Autodesk Inventor part; units mm, degrees
ref_plane "YZ Plane" through (0, 0, 0) normal (1, 0, 0) x (0, 1, 0)
ref_plane "XZ Plane" through (0, 0, 0) normal (0, 1, 0) x (-1, 0, 0)
ref_plane "XY Plane" through (0, 0, 0) normal (0, 0, 1) x (1, 0, 0)
sketch "Sketch1" plane through (0, 0, 0) normal (0, 0, 1) x (1, 0, 0)
  line L0 (0, 0) -> (10, 0)
  line L1 (10, 0) -> (10, 48.3509)
  line L2 (10, 48.3509) -> (59.1053, 20)
  line L3 (59.1053, 20) -> (59.1053, 60)
  line L4 (59.1053, 60) -> (23.094, 60)
  line L5 (23.094, 60) -> (0, 100)
  line L6 (0, 100) -> (0, 0)
  dimension "d0" = 20
  dimension "d1" = 30
  dimension "d2" = 100
  dimension "d3" = 60
  dimension "d4" = 40
  dimension "d5" = 118.2105
  dimension "d6" = 60
revolve "Revolution1" add sketch "Sketch1" angle 360 about axis through (0, 100, 0) along (0, -1, 0)
fillet "Fillet1" radius 20 1 edges at (-10, 48.3509, 0)
equation "\"ITERACOES\" = 0"
equation "\"VALORES_OTIMOS\" = 118.21054"
properties part number "Mass_otimization" material "Steel, Mild"
Could you check a few things on this model? Use its own coordinates, in mm. A direction names the side the tool comes from. Give positions to 0.01 mm unless a question says otherwise; leave off trailing zeros. Order: outer loops, then holes, each group sorted by start corner. A loop starts at its lowest first (then second) coordinate and runs counter-clockwise, first axis right, second up. Notation, with made-up numbers: (13.5, -39) -> (23.5, -39) arc R8 cw to (23.5, -25) -> close; hole circle Ø3 at (-17, 30.25). An arc over 180 degrees is marked (long way). Answer in a Markdown table with one row per item. Add a question column.
Item 1: I'm going to push flat-ended pins straight in: P1, Ø3, axis at x = 38.5, y = 24.5, coming from the +Z side; P2, Ø8, axis at y = 58, z = 15, coming from the -X side; P3, Ø10, axis at y = 34, z = 44.5, coming from the +X side. Where does each tip first touch, or does it pass through?
Item 2: Please list where these lines run through material, in increasing order: probe 1 along Z at (x, y) = (-7.5, 29); probe 2 along Z at (x, y) = (-4, 23); probe 3 along X at (y, z) = (23, 5.5).
Item 3: Imagine slicing it at A-A (y = 47). List the corners of the cut face in (x, z) for me, and give its area (3 significant figures).
Item 4: Imagine slicing it at B-B (y = 68.5). List the corners of the cut face in (x, z) for me, and give its area (3 significant figures).
Item 5: For faces 1 (the flat face through (25, 60, 1)), 2 (the flat face through (0, 0, 0)), 3 (the cylindrical face through (-2.17, 6.95, 9.76)), which set-ups out of +Z, -Z, +X, -X, +Y, -Y let a thin tool reach every point of the face, with its end or its side?
Result:
| question | item | result |
|---|---|---|
| 1 | P1 | z = 46.09 |
| 1 | P2 | x = -58.07 |
| 1 | P3 | x = 43.97 |
| 2 | probe 1 | -58.63 to -42.87, -15.38 to 15.38, 42.87 to 58.63 |
| 2 | probe 2 | -58.97 to -53.76, -11.62 to 11.62, 53.76 to 58.97 |
| 2 | probe 3 | -58.85 to -53.63, -10.99 to 10.99, 53.63 to 58.85 |
| 3 | outline | circle Ø118.21 at (0, 0) |
| 3 | area | 11,000 mm2 |
| 4 | outline | circle Ø36.37 at (0, 0) |
| 4 | area | 1,040 mm2 |
| 5 | face 1 | +Y |
| 5 | face 2 | +Z, -Z, +X, -X, -Y |
| 5 | face 3 | -Y |
